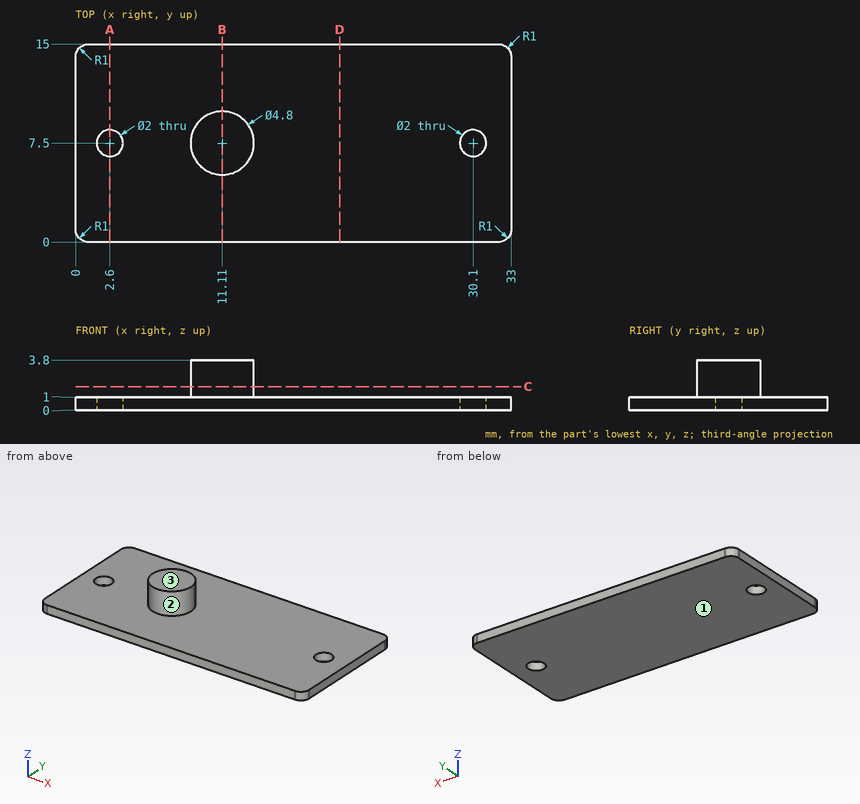
Drawing for the job (mm, zero at the part's lowest x, y, z). Coordinates: 2 decimals unless noted, no trailing zeros. Write each loop counter-clockwise with the first axis right and the second up, starting at its lowest first coordinate (ties: lowest second). Pieces come first, ordered by that corner, then holes. Notation, with made-up numbers: (13.5, 32) -> (48.5, 32) arc R17 ccw to (48.5, 45) -> close; hole circle Ø8 at (-22.75, -30). An arc over 180 degrees is marked (long way). One line per item, written item: value. Start each with the question number.
1) Slice it at D-D on x = 20. Write the cut outline in (y, z).
2) Slice it at A-A on x = 2.6. Write the cut outline in (y, z), then the cut area to 3 significant figures.
3) Flat gauge pins, fed straight in: pin 1 Ø1.5 at (x, z) = (3.5, 1.5) entering from +Y; pin 2 Ø2 at (x, y) = (9, 13) entering from +Z. Where does each tip first touch, or does it go through?
4) Slice it at B-B on x = 11.11. Write the cut outline in (y, z).
5) Probe probe 1 along Y at (x, z) = (2.6, 0.2); probe 2 along Z at (x, y) = (14, 12); probe 3 along Y at (x, z) = (29.5, 0.4). List the from-to ranges inside material, lowest first.
6) Slice it at C-C on z = 1.8. Write the cut outline in (x, y), then the cut area to 3 significant figures.
7) Pull direction Z, two halves, no side cores. Call the marked faces 1, 2 and 3: +Z half, -Z half, draft (parallel to the pull), parting line (faces both ways), or undercut.
Answers follow:
1. outline: (0, 0) -> (15, 0) -> (15, 1) -> (0, 1) -> close
2. outline: (0, 0) -> (6.5, 0) -> (6.5, 1) -> (0, 1) -> close; (8.5, 0) -> (15, 0) -> (15, 1) -> (8.5, 1) -> close
2. area: 13.0 mm2
3. pin 1: y = 15
3. pin 2: z = 1
4. outline: (0, 0) -> (15, 0) -> (15, 1) -> (9.9, 1) -> (9.9, 3.8) -> (5.1, 3.8) -> (5.1, 1) -> (0, 1) -> close
5. probe 1: 0 to 6.5, 8.5 to 15
5. probe 2: 0 to 1
5. probe 3: 0 to 6.7, 8.3 to 15
6. outline: circle Ø4.8 at (11.11, 7.5)
6. area: 18.1 mm2
7. face 1: -Z half
7. face 2: draft
7. face 3: +Z half
